```python
from build123d import *

# Parameters (mm, degrees)
BOSS_EXTRUDE2_DEPTH      = 2
SKETCH3_R                = 2
CUT_EXTRUDE1_DEPTH       = 2
BOSS_EXTRUDE3_DEPTH      = 5
BOSS_EXTRUDE3_DEPTH_BACK = 5
BOSS_EXTRUDE3_START      = -14
BOSS_EXTRUDE4_START      = -19
BOSS_EXTRUDE4_DEPTH      = 10
SKETCH5_R                = 1.5
CUT_EXTRUDE2_DEPTH       = 5
FILLET1_R                = 3
FILLET2_R                = 3


with BuildPart() as part:
    # Sketch2 → Boss-Extrude2 (new body)
    with BuildSketch(Plane(origin=(0, 0, -0.175945046), x_dir=(1, 0, 0), z_dir=(0, 1, 0))):
        Polygon((10, 12.615523277), (10, -28.082679321), (10, -35.082679321), (38, -35.082679321), (38, -28.082679321), (38, 12.615523277), (38, 19.615523277), (10, 19.615523277), align=None)
        Polygon((13, -7.733578022), (13, 12.615523277), (13, 13.615523277), (35, 13.615523277), (35, 12.615523277), (35, -7.733578022), (35, -28.082679321), (35, -29.082679321), (13, -29.082679321), (13, -28.082679321), align=None, mode=Mode.SUBTRACT)
    extrude(amount=BOSS_EXTRUDE2_DEPTH)

    # Sketch3 → Cut-Extrude1 (cut)
    with BuildSketch(Plane(origin=(0, 2, 0), x_dir=(1, 0, 0), z_dir=(0, 1, 0))):
        with Locations(Location((29, -31.707632976, 0), (0, 0, 270))):
            Circle(SKETCH3_R)
        with Locations(Location((19, -31.707632976, 0), (0, 0, 270))):
            Circle(SKETCH3_R)
        with Locations(Location((19, 16.592367024, 0), (0, 0, 270))):
            Circle(SKETCH3_R)
        with Locations(Location((29, 16.592367024, 0), (0, 0, 270))):
            Circle(SKETCH3_R)
    extrude(amount=-CUT_EXTRUDE1_DEPTH, mode=Mode.SUBTRACT)

    # Sketch4 → Boss-Extrude3 (add, two sides: drawn at the far end of the back side and taken through both)
    with BuildSketch(Plane(origin=(38, 0, 0), x_dir=(0, 0, -1), z_dir=(1, 0, 0)).offset(BOSS_EXTRUDE3_START - BOSS_EXTRUDE3_DEPTH_BACK)):
        Polygon((-34.906734274, 0), (-39.906734274, 0), (-39.906734274, 10.7), (-45.906734274, 10.7), (-45.906734274, 12.7), (-40.011651192, 12.7), (-37.906734274, 12.7), (-37.906734274, 2), (-34.906734274, 2), align=None)
    extrude(amount=BOSS_EXTRUDE3_DEPTH + BOSS_EXTRUDE3_DEPTH_BACK)

    # Sketch6 → Boss-Extrude4 (add)
    with BuildSketch(Plane(origin=(38, 0, 0), x_dir=(0, 0, -1), z_dir=(1, 0, 0)).offset(BOSS_EXTRUDE4_START)):
        Polygon((24.791468323, 0), (19.791468323, 0), (19.791468323, 2), (22.791468323, 2), (22.791468323, 12.7), (30.791468323, 12.7), (30.791468323, 10.7), (24.791468323, 10.7), align=None)
    extrude(amount=BOSS_EXTRUDE4_DEPTH)

    # Sketch5 → Cut-Extrude2 (cut)
    with BuildSketch(Plane.XZ.offset(-10.7)):
        with Locations(Location((24, -27.791468323, 0), (0, 0, 270))):
            Circle(SKETCH5_R)
        with Locations(Location((24, 42.906734274, 0), (0, 0, 270))):
            Circle(SKETCH5_R)
    extrude(amount=-CUT_EXTRUDE2_DEPTH, mode=Mode.SUBTRACT)

    # Fillet1
    fillet1_edges = [part.edges().sort_by_distance(p)[0] for p in [
        (38, 1, 34.906734274),
        (10, 1, 34.906734274),
        (10, 1, -19.791468323),
        (35, 1, 28.906734274),
        (35, 1, -13.791468323),
        (13, 1, 28.906734274),
        (13, 1, -13.791468323),
        (38, 1, -19.791468323),
        (29, 1, -19.791468323),
        (19, 1, -19.791468323),
        (19, 1, 34.906734274),
        (29, 1, 34.906734274),
    ]]
    fillet(fillet1_edges, radius=FILLET1_R)

    # Fillet2
    fillet2_edges = [part.edges().sort_by_distance(p)[0] for p in [
        (24, 0, -24.791468323),
        (24, 0, 39.906734274),
    ]]
    fillet(fillet2_edges, radius=FILLET2_R)


solid = part.part
```
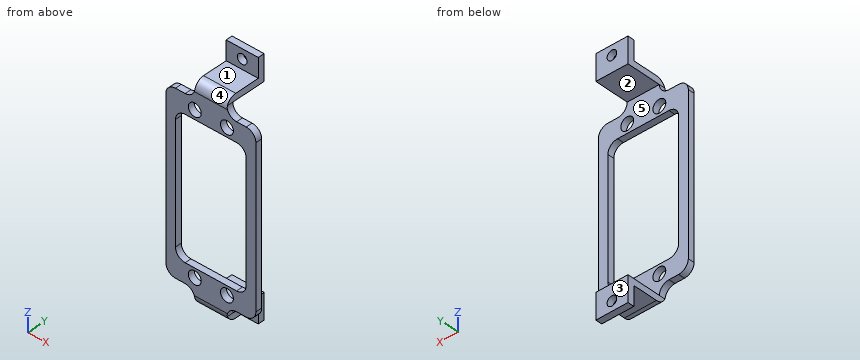
Read the model definition and answer for the solid it produces. Units are mm, in the model's axes. Face numbers are marked on the shaded views. A direction names the side the tool comes from. Give positions to 0.01 mm unless a question says otherwise; leave off trailing zeros. Write each loop counter-clockwise with the first axis right and the second up, starting at its lowest first coordinate (ties: lowest second). Pieces come first, ordered by that corner, then holes. Notation, with made-up numbers: (-39.5, -15.5) -> (7.5, -15.5) arc R9 cw to (7.5, -8.5) -> close; hole circle Ø8 at (17.25, 84). An arc over 180 degrees is marked (long way). Answer as a JSON object with one key per item and string values.
1) Section C-C on y = 5 is taken. Write down the section's boundary in (x, z).
Findings below:
{"outline": "(19, -24.79) -> (29, -24.79) -> (29, -22.79) -> (19, -22.79) -> close; (19, 37.91) -> (29, 37.91) -> (29, 39.91) -> (19, 39.91) -> close"}
2) Section D-D on y = 1 is taken. Count the separate pieces of the cut face and the enclosed holes in it, then the cut area to 3 significant figures.
Findings below:
{"separate pieces": "1", "enclosed holes": "5", "area": "634 mm^2"}
3) Section B-B on x = 24 is taken. Write down the section's boundary in (y, z), then the cut area to 3 significant figures.
Findings below:
{"outline": "(0, -21.79) arc R3 ccw to (3, -24.79) -> (10.7, -24.79) -> (10.7, -26.29) -> (12.7, -26.29) -> (12.7, -22.79) -> (2, -22.79) -> (2, -13.79) -> (0, -13.79) -> close; (0, 28.91) -> (2, 28.91) -> (2, 37.91) -> (12.7, 37.91) -> (12.7, 41.41) -> (10.7, 41.41) -> (10.7, 39.91) -> (3, 39.91) arc R3 ccw to (0, 36.91) -> close; (10.7, -30.79) -> (12.7, -30.79) -> (12.7, -29.29) -> (10.7, -29.29) -> close; (10.7, 44.41) -> (12.7, 44.41) -> (12.7, 45.91) -> (10.7, 45.91) -> close", "area": "94.9 mm^2"}
4) For a pull along Z with two mould halves and no side action, classify the marked faces 1, 2 and 3 as pulls with the +Z half, pulls with the -Z half, needs draft (parallel to the pull), parting line crosses it, or undercut.
Findings below:
{"face 1": "pulls with the +Z half", "face 2": "undercut", "face 3": "needs draft"}
5) A tool of negligible diameter and unlimited length cuts with its end or side. For the marked faces 4 and 5, from which of +Z, -Z, +X, -X, +Y, -Y can it reach the whole face along a straight path? Write none if from no direction.
Findings below:
{"face 4": "+Z, +X, -X, -Y", "face 5": "+X, -X, +Y"}
6) Flat-ended cylindrical pins translate along their axes: pin 1 Ø1.5 at (x, y) = (26.5, 7) entering from -Z; pin 2 Ø2.5 at (y, z) = (4, -25.5) entering from -X; pin 3 Ø1 at (x, z) = (13, 29) entering from +Y. Find the tip coordinate at first contact, or state that the pin passes through.
Findings below:
{"pin 1": "stops at z = -24.79", "pin 2": "stops at x = 19", "pin 3": "stops at y = 2"}
7) Section A-A on z = 0.5 is taken. Write down the section's boundary in (x, y), then the cut area to 3 significant figures.
Findings below:
{"outline": "(10, 0) -> (13, 0) -> (13, 2) -> (10, 2) -> close; (35, 0) -> (38, 0) -> (38, 2) -> (35, 2) -> close", "area": "12.0 mm^2"}
8) Straight lines are drawn through the part: probe 1 along Z at (x, y) = (24, 6.5); probe 2 along Z at (x, y) = (28, 12); probe 3 along X at (y, z) = (1, 30). For each, find the intervals that lie inside material, in ascending order. Write a range as from..to.
Findings below:
{"probe 1": "z = -24.79..-22.79, 37.91..39.91", "probe 2": "z = -30.79..-22.79, 37.91..45.91", "probe 3": "x = 10..17.96, 20.04..27.96, 30.04..38"}
